For this review, use the dimensioned drawing (mm, ordinates from the lowest corner) and the shaded views. A direction names the side the tool comes from. Coordinates: 2 decimals unless noted, no trailing zeros. Write each loop counter-clockwise with the first axis right and the second up, starting at its lowest first coordinate (ties: lowest second). Pieces come first, ordered by that corner, then holes. Notation, with made-up numbers: (-6, -7.5) - (47, -7.5) arc R27 cw to (47, 17.5) - close; hole circle Ø4 at (50, 18). An arc over 180 degrees is marked (long way). One line per item, written item: value.
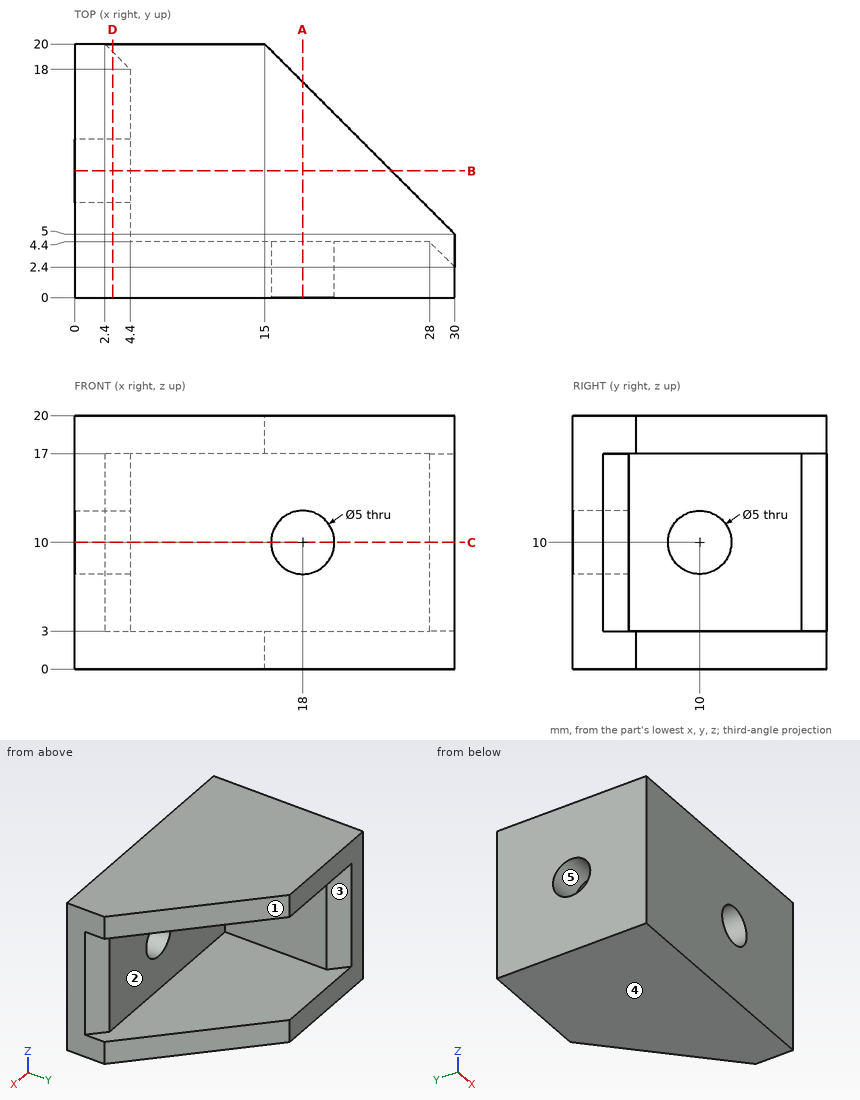
1. Consider section B-B, the plane y = 10. Write out the cut boundary in (x, z).
Answer block:
outline: (0, 0) - (25, 0) - (25, 3) - (4.4, 3) - (4.4, 7.5) - (0, 7.5) - close; (0, 12.5) - (4.4, 12.5) - (4.4, 17) - (25, 17) - (25, 20) - (0, 20) - close
2. Mouldability with a two-part tool opening along Y and no side actions: class the marked faces 3, 4 and 5 as released by +Y, released by -Y, zero draft, split by the parting line, or undercut.
Answer block:
face 3: released by +Y
face 4: zero draft
face 5: undercut
3. Insertion check: pin 1 Ø5 at (x, z) = (25, 7) entering from +Y; pin 2 Ø5.5 at (x, y) = (19.5, 12.5) entering from -Z; pin 3 Ø8 at (x, z) = (24, 2) entering from +Y; pin 4 Ø4.5 at (y, z) = (10, 10) entering from -X. Each pin has a flat end and moves straight along its axis. Give the tip position at first contact, or say it passes through.
Answer block:
pin 1: stops at y = 4.4
pin 2: stops at z = 0
pin 3: stops at y = 15
pin 4: passes through
4. Consider section D-D, the plane x = 3. Write out the cut boundary in (y, z), then the cut area to 3 significant figures.
Answer block:
outline: (0, 0) - (20, 0) - (20, 3) - (19.4, 3) - (19.4, 17) - (20, 17) - (20, 20) - (0, 20) - close; hole circle Ø5 at (10, 10)
area: 372 mm^2
5. Consider section A-A, the plane x = 18. Write out the cut boundary in (y, z).
Answer block:
outline: (0, 0) - (17, 0) - (17, 3) - (4.4, 3) - (4.4, 7.5) - (0, 7.5) - close; (0, 12.5) - (4.4, 12.5) - (4.4, 17) - (17, 17) - (17, 20) - (0, 20) - close
6. Wall thickness on line 1 along Z through (x, y) = (5.25, 7.25); line 2 along Y through (x, z) = (2.25, 10): over which ranges is each line inside the solid? List them lowest first.
Answer block:
line 1: z = 0 to 3, 17 to 20
line 2: y = 0 to 7.5, 12.5 to 20
7. For the marked faces 1 and 2, list the 3-axis set-ups (+Z, -Z, +X, -X, +Y, -Y) from which the entire face can be reached by the end or side of a thin tool; tool diameter is ignored.
Answer block:
face 1: +Z, -Z, +X, +Y
face 2: +X, +Y
8. Consider section C-C, the plane z = 10. Write out the cut boundary in (x, y), then the cut area to 3 significant figures.
Answer block:
outline: (0, 0) - (15.5, 0) - (15.5, 4.4) - (4.4, 4.4) - (4.4, 7.5) - (0, 7.5) - close; (0, 12.5) - (4.4, 12.5) - (4.4, 18) - (2.4, 20) - (0, 20) - close; (20.5, 0) - (30, 0) - (30, 2.4) - (28, 4.4) - (20.5, 4.4) - close
area: 153 mm^2
